Geometry check sheet. Reference: the model listing, model coordinates, mm. A direction names the side the tool comes from. Coordinates: 2 decimals unless noted, no trailing zeros. Loops run counter-clockwise (first coordinate to the right, second up) from the corner with the lowest first, then second, coordinate; pieces in that order, holes last. Notation, with made-up numbers: (-12.75, -30.5) -> (1.25, -30.5) arc R22 cw to (1.25, -14.5) -> close; hole circle Ø6 at (-37.75, 43). An arc over 180 degrees is marked (long way). Answer as a JSON object with one key per item and string values.
from build123d import *

# Parameters (mm, degrees)
F1_DEPTH = 24
F2_T     = -1.5
F3_R     = 5
F4_DEPTH = 5
F5_R     = 7.5
F6_DEPTH = 5


with BuildPart() as f1:
    # F0 (on Right) → F1 (new body)
    with BuildSketch(Plane.YZ):
        with BuildLine():
            Line((8.7272727273, -30), (8.7272727273, -10))
            ThreePointArc((8.7272727273, -10), (5.4922936244, 12.0830459736), (-13.2727272727, 0))
            Line((-13.2727272727, 0), (-13.2727272727, -42))
            Line((-13.2727272727, -42), (16.7272727273, -42))
            Line((16.7272727273, -42), (16.7272727273, -30))
            Line((16.7272727273, -30), (8.7272727273, -30))
        make_face()
    extrude(amount=F1_DEPTH)

    # F2
    f2_openings = [f1.faces().sort_by_distance(p)[0] for p in [
        (12, 1.727273, -42),
    ]]
    offset(amount=F2_T, openings=f2_openings, kind=Kind.INTERSECTION)

    # F3 (on face) → F4 (cut)
    with BuildSketch(Plane(origin=(0, 0, 0), x_dir=(0, -1, 0), z_dir=(-1, 0, 0))):
        Circle(F3_R)
    extrude(amount=-F4_DEPTH, mode=Mode.SUBTRACT)

    # F5 (on face) → F6 (cut)
    with BuildSketch(Plane.XZ.offset(13.2727272727)):
        with Locations((12, -10)):
            Circle(F5_R)
        with Locations((12, -30)):
            Circle(F5_R)
    extrude(amount=-F6_DEPTH, mode=Mode.SUBTRACT)


with BuildPart() as f7_1:
    # F7: instance of F1
    add(f1.part.mirror(Plane(origin=(0, -0.4359832268, -17.1422397222), x_dir=(0, 1, 0), z_dir=(-1, 0, 0))))


solid = f7_1.part
1. Section check A-A, the plane x = -12. Record the boundary of the cut face in (y, z).
Evaluation:
{"outline": "(-13.27, -42) -> (-11.77, -42) -> (-11.77, -37.5) -> (-13.27, -37.5) -> close; (-13.27, -22.5) -> (-11.77, -22.5) -> (-11.77, -17.5) -> (-13.27, -17.5) -> close; (-13.27, -2.5) -> (-11.77, -2.5) -> (-11.77, 0) arc R11.77 cw (long way) to (7.23, -9.29) -> (7.23, -31.5) -> (15.23, -31.5) -> (15.23, -42) -> (16.73, -42) -> (16.73, -30) -> (8.73, -30) -> (8.73, -10) arc R13.27 ccw (long way) to (-13.27, 0) -> close"}
2. Thickness scan on probe 1 along Y at (x, z) = (-19.5, -36); probe 2 along Y at (x, z) = (-3.5, -27); probe 3 along X at (y, z) = (-3, -6.5). Record the ranges inside material, lowest first. Write a range as from..to.
Evaluation:
{"probe 1": "y = -13.27..-11.77, 15.23..16.73", "probe 2": "y = -13.27..-11.77, 7.23..8.73", "probe 3": "x = -24..-22.5, -1.5..0"}
3. Depth check by flat-ended pin: P1, Ø12, axis at x = -12, z = -10, coming from the +Y side; P2, Ø8, axis at y = 7, z = -3.5, coming from the +X side; P3, Ø1.5, axis at x = -8, y = 11, coming from the +Z side; P4, Ø1.5, axis at x = -11, z = -30, coming from the -Y side. Enter the tip coordinate at first touch or a pass-through.
Evaluation:
{"P1": "stops at y = 12.66", "P2": "stops at x = 0", "P3": "stops at z = 8.43", "P4": "stops at y = 7.23"}
4. Section check B-B, the plane z = -18.5. Record the boundary of the cut face in (x, y), then the cut area to 3 significant figures.
Evaluation:
{"outline": "(-24, -13.27) -> (0, -13.27) -> (0, 8.73) -> (-24, 8.73) -> close; hole (-22.5, -11.77) -> (-1.5, -11.77) -> (-1.5, 7.23) -> (-22.5, 7.23) -> close", "area": "129 mm^2"}
5. Section check D-D, the plane x = -3.75. Record the boundary of the cut face in (y, z).
Evaluation:
{"outline": "(-13.27, -42) -> (-11.77, -42) -> (-11.77, 0) arc R11.77 cw (long way) to (7.23, -9.29) -> (7.23, -31.5) -> (15.23, -31.5) -> (15.23, -42) -> (16.73, -42) -> (16.73, -30) -> (8.73, -30) -> (8.73, -10) arc R13.27 ccw (long way) to (-13.27, 0) -> close"}
6. Mould release check, pull along Y, two halves, no side actions. Record for faces 6 (the face through (-11.853, 5.47, 10.425)), 7 (the face through (-12, 15.227, -37)), 8 (the face through (-10.37, -12.53, -37.32)), 9 (the face through (-12, 16.727, -36)): released by +Y, released by -Y, zero draft, split by the parting line, or undercut.
Evaluation:
{"face 6": "undercut", "face 7": "undercut", "face 8": "zero draft", "face 9": "released by +Y"}
7. Section check C-C, the plane y = 10. Record the boundary of the cut face in (x, z), then the cut area to 3 significant figures.
Evaluation:
{"outline": "(-24, -42) -> (-22.5, -42) -> (-22.5, -31.5) -> (-1.5, -31.5) -> (-1.5, -42) -> (0, -42) -> (0, -30) -> (-24, -30) -> close; (-24, -8.73) -> (0, -8.73) -> (0, 8.73) -> (-24, 8.73) -> close; hole (-22.5, -6.21) -> (-1.5, -6.21) -> (-1.5, 6.21) -> (-22.5, 6.21) -> close", "area": "225 mm^2"}
8. Tool access check on faces 1 (the face through (-10.37, -12.53, -17.32)), 2 (the face through (-12, 13, -30)), 3 (the face through (-23, 1, -42)), 4 (the face through (-0.74, 1.08, -4.88)), 5 (the face through (-12, -11.773, -21)). Record the directions out of +Z, -Z, +X, -X, +Y, -Y that give a thin tool (end or side, any length) a straight path to the whole face; none if there is none.
Evaluation:
{"face 1": "-Y", "face 2": "+X, -X, +Y", "face 3": "-Z, +X, -X, +Y, -Y", "face 4": "+X", "face 5": "-Z"}
